Autodesk Inventor part; units mm, degrees
ref_plane "YZ Plane" through (0, 0, 0) normal (1, 0, 0) x (0, 1, 0)
ref_plane "XZ Plane" through (0, 0, 0) normal (0, 1, 0) x (-1, 0, 0)
ref_plane "XY Plane" through (0, 0, 0) normal (0, 0, 1) x (1, 0, 0)
sketch "Sketch1" plane through (0, 0, 0) normal (0, 1, 0) x (-1, 0, 0)
  circle A0 centre (0, 0) radius 27.25
  circle A1 centre (0, 0) radius 40
  line L0 (0, 40) -> (0, -40)
  line L1 (0, 27.25) -> (0, 40)
  line L2 (0, 0) -> (45.8367, 0)
  line L3 (0, -27.25) -> (0, -40)
  circle A2 centre (0, 0) radius 35
  line L4 (0, -27.25) -> (10, -27.25)
  line L5 (10, -27.25) -> (10, -40)
  line L6 (10, -40) -> (0, -40)
  line L7 (0, -40) -> (0, -27.25)
  line L8 (0, 27.25) -> (10, 27.25)
  line L9 (10, 27.25) -> (10, 40)
  line L10 (10, 40) -> (0, 40)
  point P0 (0, -26.75)
  point P1 (0, 35)
  point P2 (0, -35)
  point P3 (10, -33.541)
  point P4 (10, 38.7298)
  point P5 (10, 33.541)
  dimension "d0" = 54.5
  dimension "d1" = 80
  dimension "d15" = 70
  dimension "d18" = 10
extrude "Extrusion6" add sketch "Sketch1" along normal blind 10 contours A2 L9 A1 L2 | L2 A1 L5 A2 | L0 A1 L9 A2 | A2 L5 A1 L0
extrude "Extrusion7" add sketch "Sketch1" along normal blind 19 contours L2 A2 L5 L4 A0 | A0 L8 L9 A2 L2 | L0 A2 L9 L8 | L4 L5 A2 L0 | L0 A1 L9 A2 | A2 L5 A1 L0 | L10 L9 A1 | A1 L5 L6
chamfer "Chamfer1" distance 10 distance2 1.25 1 edges at (-10, 9.5, -40) measured on face at (-3.3333, 6.3333, -40)
chamfer "Chamfer2" distance 1.25 distance2 10 1 edges at (-10, 9.5, 40) measured on face at (-10, 16, 37.4236)
chamfer "Chamfer3" distance 6.75 distance2 9 1 edges at (-35, 19, 0) measured on face at (-3.3335, 19, -33.597)
chamfer "Chamfer4" distance 3 distance2 3.5 1 edges at (-40, 10, 0) measured on face at (-36.5086, 10, 0)
fillet "Fillet1" radius 3 2 edges at (-5.0003, 19, 39.3753) (-5.0003, 19, -39.3753)
sketch "Sketch3" plane through (-10, 0, -38.7298) normal (-1, 0, 0) x (0, 0, 1)
  line L0 (-0.0202, 0) -> (-0.0202, 16)
  line L1 (-0.0202, 14.7921) -> (4.9798, 14.7921)
  line L2 (4.9798, 14.7921) -> (4.9798, 19.7921)
  circle A0 centre (4.9798, 14.7921) radius 0.25
  point P0 (38.7298, 0)
  dimension "d32" = 5
  dimension "d33" = 5
  dimension "d34" = 0.5
extrude "Extrusion8" cut sketch "Sketch3" against normal through all
mirror "Mirror1" about plane through (0, 0, 0) normal (0, 0, 1) of "Extrusion8"
properties part number "Obrecz_kolanko"
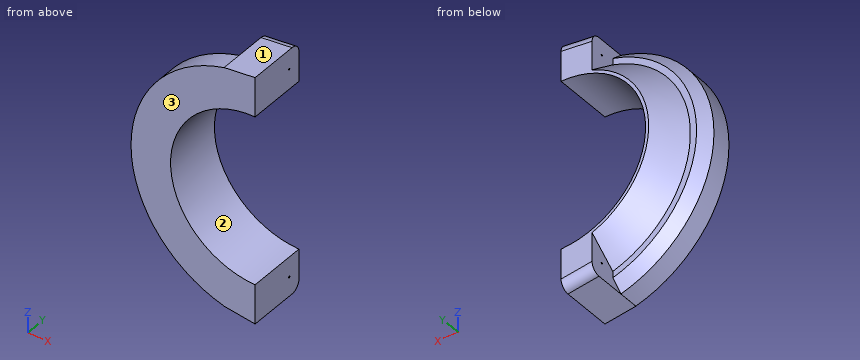
Model file for the job. Use its own axes, mm. Face numbers are marked on the shaded views. Round coordinates to 2 decimals unless told otherwise and drop trailing zeros. Answer as CSV lines item,"result". Start each with the question number.
1) Mould opens along Z. For the marked faces 1, 2 and 3 say: +Z half, -Z half, draft (parallel to the pull), parting line (faces both ways), or undercut.
2) Slice it at C-C (x = -4). State how many separate pieces and enclosed holes the cut face has, plus the area to 3 significant figures.
3) Pin check, flat tips, straight feed: P1, Ø6, axis at x = -30.5, y = 6.5, coming from the +Z side; P2, Ø3, axis at y = 6.5, z = 15.5, coming from the +X side; P3, Ø10, axis at y = 13, z = 35, coming from the -X side. Stop position of each tip, or through.
4) Probe line 1 along Y through (x, z) = (-2.25, -33.75); line 2 along X through (y, z) = (16.5, -32.5); line 3 along Z through (x, y) = (-25, 6.5). List the from-to ranges inside material, lowest first.
Filled in:
1,face 1,"+Z half"
1,face 2,"undercut"
1,face 3,"draft"
2,separate pieces,"2"
2,enclosed holes,"2"
2,area,"472 mm2"
3,P1,"stops at z = 29.05"
3,P2,"stops at x = -21.3"
3,P3,"stops at x = -20.33"
4,line 1,"y = 0 to 14.54, 15.04 to 19"
4,line 2,"x = -10 to 0"
4,line 3,"z = -31.22 to -10.84, 10.84 to 31.22"
